Input: part model. Units: mm. Frame: model coordinates. Face numbers are marked on the shaded views. A direction names the side the tool comes from. Coordinates: 2 decimals unless noted, no trailing zeros. Loops run counter-clockwise (first coordinate to the right, second up) from the corner with the lowest first, then second, coordinate; pieces in that order, holes last. Notation, with made-up numbers: (82, -26.5) -> (97, -26.5) arc R17 ccw to (97, -16.5) -> close; hole circle Ø9 at (75.25, 79). An arc over 180 degrees is marked (long way). Put each result on its own line as item: value. Start each with the question number.
1) Cut plane D-D (z = 2.5). Return the cut outline in (x, y), plus the area to 3 significant figures.
2) Cut plane A-A (x = 41). Return the cut outline in (y, z).
3) Cut plane C-C (y = 23.75). Return the cut outline in (x, z), plus the area to 3 significant figures.
4) Contact query for flat-ended pins moving along their axis: P1, Ø15, axis at x = 50, y = 12, coming from the -Z side; P2, Ø1.6, axis at y = 16, z = 35, coming from the -X side; P3, Ø0.6, axis at y = 12, z = 39, coming from the -X side. Output: stop coordinate, or through.
5) Pull-direction query (Z, two-part tool) for the marked faces 3, 4 and 5; classes: pulls with the +Z half, pulls with the -Z half, needs draft (parallel to the pull), parting line crosses it, or undercut.
6) Set-up query: the marked faces 1 and 2. Return all of +Z, -Z, +X, -X, +Y, -Y with unobstructed straight access to the full face (end or side cutting, diameter ignored); none if empty.
7) Material intervals for L1, parallel to Y at x = 47, z = 2.8; L2, parallel to Z at x = 63, y = 27; L3, parallel to Y at x = 52.5, z = 19, sorted ascending.
8) Cut plane B-B (x = 67). State how many separate pieces and enclosed holes the cut face has, plus the area to 3 significant figures.
from build123d import *

# Parameters (mm, degrees)
SKETCH1_W           = 79
SKETCH1_H           = 37.5
SKETCH1_R           = 2
BODY_DEPTH          = 5
SKETCH2_W           = 79
SKETCH2_H           = 4
LEG1_DEPTH          = 3
SKETCH3_W           = 4
SKETCH3_H           = 4
LEG2_DEPTH          = 3
SKETCH4_W           = 79
SKETCH4_H           = 4
LEG3_DEPTH          = 3
WALLS_DEPTH         = 33
SKETCH6_W           = 2
SKETCH6_H           = 34.5
CUT_EXTRUDE1_DEPTH  = 17
SKETCH7_W           = 73
SKETCH7_H           = 37.5
BOSS_EXTRUDE1_DEPTH = 3
FILLET1_R           = 1
FILLET2_R           = 1
FILLET3_R           = 1
FILLET4_R           = 1
FILLET6_R           = 1
SKETCH8_W           = 5
SKETCH8_H           = 31.5
BOSS_EXTRUDE2_DEPTH = 16


with BuildPart() as part:
    # Sketch1 → Body (new body)
    with BuildSketch(Plane.XY):
        with Locations((39.5, 18.75)):
            Rectangle(SKETCH1_W, SKETCH1_H)
        with Locations((47, 23.75)):
            Circle(SKETCH1_R, mode=Mode.SUBTRACT)
        with Locations((32, 23.75)):
            Circle(SKETCH1_R, mode=Mode.SUBTRACT)
        with Locations((32, 13.75)):
            Circle(SKETCH1_R, mode=Mode.SUBTRACT)
        with Locations((47, 13.75)):
            Circle(SKETCH1_R, mode=Mode.SUBTRACT)
    extrude(amount=BODY_DEPTH)

    # Sketch2 → Leg1 (add)
    with BuildSketch(Plane(origin=(0, 0, 0), x_dir=(-1, 0, 0), z_dir=(0, 0, -1))):
        with Locations((-39.5, 35.5)):
            Rectangle(SKETCH2_W, SKETCH2_H)
        with Locations((-39.5, 2)):
            Rectangle(SKETCH2_W, SKETCH2_H)
    extrude(amount=LEG1_DEPTH)

    # Sketch3 → Leg2 (add)
    with BuildSketch(Plane(origin=(0, 0, -3), x_dir=(-1, 0, 0), z_dir=(0, 0, -1))):
        with Locations((-77, 35.5)):
            Rectangle(SKETCH3_W, SKETCH3_H)
        with Locations((-2, 35.5)):
            Rectangle(SKETCH3_W, SKETCH3_H)
        with Locations((-2, 2)):
            Rectangle(SKETCH3_W, SKETCH3_H)
        with Locations((-77, 2)):
            Rectangle(SKETCH3_W, SKETCH3_H)
    extrude(amount=LEG2_DEPTH)

    # Sketch4 → Leg3 (add)
    with BuildSketch(Plane(origin=(0, 0, -6), x_dir=(-1, 0, 0), z_dir=(0, 0, -1))):
        with Locations((-39.5, 35.5)):
            Rectangle(SKETCH4_W, SKETCH4_H)
        with Locations((-39.5, 2)):
            Rectangle(SKETCH4_W, SKETCH4_H)
    extrude(amount=LEG3_DEPTH)

    # Sketch5 → Walls (add)
    with BuildSketch(Plane.XY.offset(5)):
        Polygon((0, 37.5), (79, 37.5), (79, 34.5), (79, 29.685442104), (79, 7.814557896), (79, 3), (79, 0), (0, 0), (0, 3), (3, 3), (76, 3), (76, 34.5), (3, 34.5), (0, 34.5), align=None)
    extrude(amount=WALLS_DEPTH)

    # Sketch6 → Cut-Extrude1 (cut)
    with BuildSketch(Plane.XY.offset(38)):
        with Locations((4.5, 18.75)):
            Rectangle(SKETCH6_W, SKETCH6_H)
    extrude(amount=-CUT_EXTRUDE1_DEPTH, mode=Mode.SUBTRACT)

    # Sketch7 → Boss-Extrude1 (add)
    with BuildSketch(Plane.XY.offset(38)):
        with Locations((42.5, 18.75)):
            Rectangle(SKETCH7_W, SKETCH7_H)
    extrude(amount=BOSS_EXTRUDE1_DEPTH)

    # Fillet1
    fillet1_edges = [part.edges().sort_by_distance(p)[0] for p in [
        (39.5, 37.5, -9),
    ]]
    fillet(fillet1_edges, radius=FILLET1_R)

    # Fillet2
    fillet2_edges = [part.edges().sort_by_distance(p)[0] for p in [
        (39.5, 33.5, -9),
    ]]
    fillet(fillet2_edges, radius=FILLET2_R)

    # Fillet3
    fillet3_edges = [part.edges().sort_by_distance(p)[0] for p in [
        (39.5, 0, -9),
    ]]
    fillet(fillet3_edges, radius=FILLET3_R)

    # Fillet4
    fillet4_edges = [part.edges().sort_by_distance(p)[0] for p in [
        (39.5, 4, -9),
    ]]
    fillet(fillet4_edges, radius=FILLET4_R)

    # Fillet6
    fillet6_edges = [part.edges().sort_by_distance(p)[0] for p in [
        (79, 2, -9),
        (79, 3.707106781, -8.707106781),
        (79, 0.292893219, -8.707106781),
        (79, 4, -4),
        (79, 0, 16.5),
        (79, 18.75, 0),
        (79, 18.75, 41),
        (79, 33.5, -4),
        (79, 37.5, 16.5),
        (79, 33.792893219, -8.707106781),
        (79, 37.207106781, -8.707106781),
        (79, 35.5, -9),
        (0, 2, -9),
        (0, 3.707106781, -8.707106781),
        (0, 0.292893219, -8.707106781),
        (0, 4, -4),
        (0, 0, 15),
        (42.5, 0, 41),
        (0, 18.75, 0),
        (42.5, 37.5, 41),
        (6, 18.75, 41),
        (0, 33.5, -4),
        (0, 37.5, 15),
        (0, 33.792893219, -8.707106781),
        (0, 37.207106781, -8.707106781),
        (0, 35.5, -9),
        (0, 1.5, 38),
        (0, 3, 21.5),
        (0, 18.75, 5),
        (0, 34.5, 21.5),
        (0, 36, 38),
    ]]
    fillet(fillet6_edges, radius=FILLET6_R)

    # Sketch8 → Boss-Extrude2 (add)
    with BuildSketch(Plane.ZY.offset(-76)):
        with Locations((30, 18.75)):
            Rectangle(SKETCH8_W, SKETCH8_H)
    extrude(amount=BOSS_EXTRUDE2_DEPTH)


solid = part.part
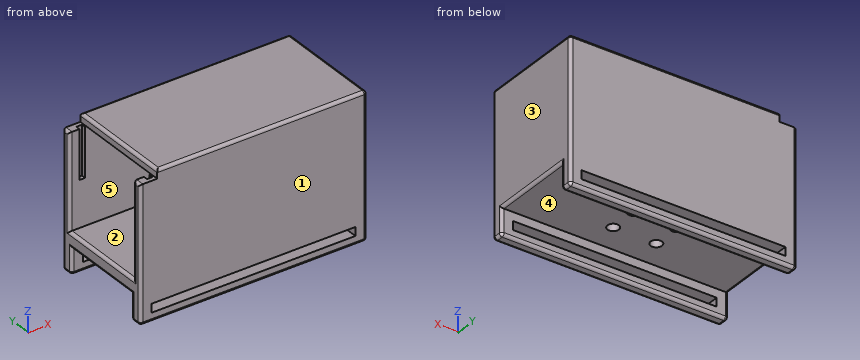
Results found:
1. outline: (0, 1) arc R1 ccw to (1, 0) -> (78, 0) arc R1 ccw to (79, 1) -> (79, 36.5) arc R1 ccw to (78, 37.5) -> (1, 37.5) arc R1 ccw to (0, 36.5) -> close; hole circle Ø4 at (32, 13.75); hole circle Ø4 at (32, 23.75); hole circle Ø4 at (47, 13.75); hole circle Ø4 at (47, 23.75)
1. area: 2,910 mm2
2. outline: (0, -8) arc R1 ccw to (1, -9) -> (3, -9) arc R1 ccw to (4, -8) -> (4, -6) -> (0, -6) -> close; (0, -3) -> (4, -3) -> (4, 0) -> (33.5, 0) -> (33.5, -3) -> (37.5, -3) -> (37.5, 40) arc R1 ccw to (36.5, 41) -> (1, 41) arc R1 ccw to (0, 40) -> close; (33.5, -8) arc R1 ccw to (34.5, -9) -> (36.5, -9) arc R1 ccw to (37.5, -8) -> (37.5, -6) -> (33.5, -6) -> close; hole (3, 5) -> (34.5, 5) -> (34.5, 38) -> (3, 38) -> close
3. outline: (0, 1) arc R1 ccw to (1, 0) -> (30, 0) -> (30, 5) -> (1, 5) arc R1 ccw to (0, 4) -> close; (6, 38) -> (76, 38) -> (76, 32.5) -> (60, 32.5) -> (60, 27.5) -> (76, 27.5) -> (76, 5) -> (49, 5) -> (49, 0) -> (78, 0) arc R1 ccw to (79, 1) -> (79, 40) arc R1 ccw to (78, 41) -> (7, 41) arc R1 ccw to (6, 40) -> close; (34, 0) -> (45, 0) -> (45, 5) -> (34, 5) -> close
3. area: 752 mm2
4. P1: stops at z = 0
4. P2: stops at x = 76
4. P3: stops at x = 6
5. face 3: needs draft
5. face 4: pulls with the -Z half
5. face 5: undercut
6. face 1: +Z, -Z, +X, -X, -Y
6. face 2: -X
7. L1: y = 0 to 11.75, 15.75 to 21.75, 25.75 to 37.5
7. L2: z = 0 to 5, 27.5 to 32.5, 38 to 41
7. L3: y = 0 to 3, 34.5 to 37.5
8. separate pieces: 3
8. enclosed holes: 2
8. area: 702 mm2
